Here's how the part is built. I have some questions about the finished solid (model axes, mm). A direction names the side the tool comes from. Round coordinates to 2 decimals unless told otherwise and drop trailing zeros. Write each loop counter-clockwise with the first axis right and the second up, starting at its lowest first coordinate (ties: lowest second). Pieces come first, ordered by that corner, then holes. Notation, with made-up numbers: (30.5, -29) - (68.5, -29) arc R33 ccw to (68.5, -1) - close; hole circle Ø10 at (72.5, 84.25). An arc over 180 degrees is marked (long way). One line per question, with ' | ' between items. Start each with the question number.
(1) Thinking about a two-plate mould opening in X: for faces 1 (the flat face through (177.8, -205, -13)), 2 (the flat face through (25.4, -206, -13)), 3 (the flat face through (228.6, -201, -13)), 4 (the flat face through (240, -201, -25.4)), which applies, pulls with the +X half, pulls with the -X half, needs draft (parallel to the pull), parting line crosses it, or undercut?
(2) Imagine slicing it at B-B (y = -314). Write out the boundary of the cut face in (x, z), plus the area to 3 significant figures.
(3) For faces 5 (the flat face through (204, -330.2, -13)), 6 (the flat face through (381, -201, -13)), which set-ups out of +Z, -Z, +X, -X, +Y, -Y let a thin tool reach every point of the face, with its end or its side?
(4) If I drill on L1, parallel to X at y = -150.5, z = -5.5, over which ranges is the centre line in solid material (lowest first)?
(5) Imagine slicing it at C-C (x = 183). Write out the boundary of the cut face in (y, z), plus the area to 3 significant figures.
(6) Imagine slicing it at A-A (z = -6). Write out the boundary of the cut face in (x, y).
(7) Will this pin go through, and if not, where does the flat tip stop? pin 1 (6 mm diameter, centred on x = 329, y = -159, fed in from +Z).
Autodesk Inventor part; units mm, degrees
ref_plane "YZ Plane" through (0, 0, 0) normal (1, 0, 0) x (0, 1, 0)
ref_plane "XZ Plane" through (0, 0, 0) normal (0, 1, 0) x (-1, 0, 0)
ref_plane "XY Plane" through (0, 0, 0) normal (0, 0, 1) x (1, 0, 0)
sketch "Sketch1" plane through (0, 0, 0) normal (0, 0, 1) x (1, 0, 0)
  line L0 (0, 0) -> (812.8, 0) construction
  line L1 (812.8, 0) -> (812.8, -406.4) construction
  line L2 (812.8, -406.4) -> (0, -406.4) construction
  line L3 (0, -406.4) -> (0, 0) construction
  line L4 (0, 0) -> (406.4, 0)
  line L5 (406.4, 0) -> (406.4, -25.4)
  line L6 (406.4, -25.4) -> (0, -25.4)
  line L7 (0, -25.4) -> (0, 0)
  line L8 (406.4, -25.4) -> (381, -25.4)
  line L9 (381, -25.4) -> (381, -406.4)
  line L10 (381, -406.4) -> (406.4, -406.4)
  line L11 (406.4, -406.4) -> (406.4, -25.4)
  line L12 (381, -406.4) -> (0, -406.4)
  line L13 (0, -406.4) -> (0, -381)
  line L14 (0, -381) -> (381, -381)
  line L15 (381, -381) -> (381, -406.4)
  line L16 (0, -381) -> (25.4, -381)
  line L17 (25.4, -381) -> (25.4, -25.4)
  line L18 (25.4, -25.4) -> (0, -25.4)
  line L19 (0, -25.4) -> (0, -381)
  dimension "d1" = 812.8
  dimension "d5" = 406.4
  dimension "d6" = 25.4
  dimension "d7" = 25.4
  dimension "d8" = 381
  dimension "d9" = 381
  dimension "d10" = 25.4
  dimension "d11" = 25.4
extrude "Extrusion1" add sketch "Sketch1" against normal blind 25.4 contours L6 L9 L14 L17
sketch "Sketch3" plane through (0, 0, 0) normal (0, 0, 1) x (1, 0, 0)
  line L0 (-406.4, 0) -> (406.4, 0) construction
  line L1 (406.4, 0) -> (406.4, -406.4) construction
  line L2 (406.4, -406.4) -> (-406.4, -406.4) construction
  line L3 (-406.4, -406.4) -> (-406.4, 0) construction
  line L4 (406.4, 0) -> (406.4, -406.4)
  line L5 (381, -381) -> (25.4, -381)
  line L6 (203.2, -381) -> (203.2, -355.6)
  line L7 (203.2, -355.6) -> (254, -355.6)
  line L8 (254, -355.6) -> (254, -50.8)
  line L9 (254, -50.8) -> (152.4, -50.8)
  line L10 (152.4, -50.8) -> (152.4, -355.6)
  line L11 (152.4, -355.6) -> (203.2, -355.6)
  point P0 (0, 0)
  dimension "d36" = 812.8
  dimension "d45" = 25.4
  dimension "d46" = 50.8
  dimension "d47" = 304.8
  dimension "d48" = 101.6
extrude "Extrusion3" cut sketch "Sketch3" against normal blind 25.4
sketch "Sketch4" plane through (0, 0, 0) normal (0, 0, 1) x (1, 0, 0)
  line L0 (152.4, -50.8) -> (152.4, -355.6)
  line L1 (152.4, -50.8) -> (177.8, -50.8)
  line L2 (177.8, -50.8) -> (177.8, -76.2)
  line L3 (177.8, -76.2) -> (152.4, -76.2)
  line L4 (152.4, -76.2) -> (152.4, -50.8)
  line L5 (254, -355.6) -> (254, -50.8)
  line L6 (254, -355.6) -> (228.6, -355.6)
  line L7 (228.6, -355.6) -> (228.6, -330.2)
  line L8 (228.6, -330.2) -> (254, -330.2)
  line L9 (254, -330.2) -> (254, -355.6)
  line L10 (228.6, -330.2) -> (177.8, -330.2)
  line L11 (177.8, -330.2) -> (177.8, -76.2)
  line L12 (177.8, -76.2) -> (228.6, -76.2)
  line L13 (228.6, -76.2) -> (228.6, -330.2)
  line L14 (152.4, -50.8) -> (254, -50.8)
  line L15 (254, -50.8) -> (254, -355.6)
  line L16 (254, -355.6) -> (152.4, -355.6)
  line L17 (152.4, -355.6) -> (152.4, -50.8)
  point P0 (0, 0)
  dimension "d51" = 25.4
  dimension "d52" = 25.4
  dimension "d53" = 25.4
  dimension "d54" = 25.4
extrude "Extrusion4" add sketch "Sketch4" against normal blind 25.4 contours L1 L2 L3 L0 | L3 L11 L10 L7 L16 L0 | L14 L5 L8 L13 L12 L2 | L7 L8 L5 L6
properties part number "JukeBox Top Panel SQ" material "Oak, Red"
Check sheet entries:
1) face 1: undercut | face 2: pulls with the -X half | face 3: undercut | face 4: needs draft
2) outline: (25.4, -25.4) - (177.8, -25.4) - (177.8, 0) - (25.4, 0) - close; (228.6, -25.4) - (381, -25.4) - (381, 0) - (228.6, 0) - close | area: 7,740 mm^2
3) face 5: +Z, -Z | face 6: +Z, -Z, +X, +Y, -Y
4) L1: 25.4 to 177.8, 228.6 to 381
5) outline: (-381, -25.4) - (-330.2, -25.4) - (-330.2, 0) - (-381, 0) - close; (-76.2, -25.4) - (-25.4, -25.4) - (-25.4, 0) - (-76.2, 0) - close | area: 2,580 mm^2
6) outline: (25.4, -381) - (381, -381) - (381, -25.4) - (25.4, -25.4) - close; hole (177.8, -330.2) - (228.6, -330.2) - (228.6, -76.2) - (177.8, -76.2) - close
7) pin 1: z = 0
